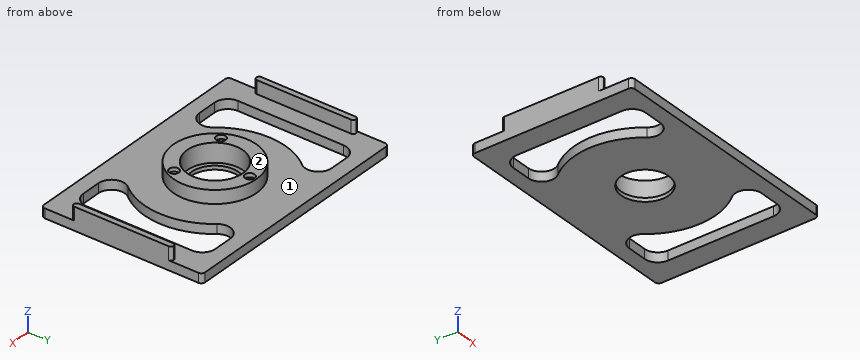
Autodesk Inventor part; units mm, degrees
ref_plane "YZ Plane" through (0, 0, 0) normal (1, 0, 0) x (0, 1, 0)
ref_plane "XZ Plane" through (0, 0, 0) normal (0, 1, 0) x (-1, 0, 0)
ref_plane "XY Plane" through (0, 0, 0) normal (0, 0, 1) x (1, 0, 0)
sketch "Skizze1" plane through (0, 0, 0) normal (0, 0, 1) x (1, 0, 0)
  line L0 (0, 0) -> (127.5, 0)
  line L1 (127.5, 0) -> (127.5, -85.5)
  line L2 (127.5, -85.5) -> (0, -85.5)
  line L3 (0, -85.5) -> (0, 0)
  dimension "d0" = 127.5
  dimension "d1" = 85.5
extrude "Extrusion1" add sketch "Skizze1" along normal blind 5
sketch "Skizze2" plane through (0, 0, 5) normal (0, 0, 1) x (1, 0, 0)
  line L0 (0, -16.25) -> (3, -16.25)
  line L1 (3, -16.25) -> (3, -69.25)
  line L2 (3, -69.25) -> (0, -69.25)
  line L3 (0, -69.25) -> (0, -16.25)
  line L4 (63.75, 42.9175) -> (63.75, -147.2432)
  line L5 (127.5, -85.5) -> (127.5, 0)
  line L6 (127.5, -16.25) -> (124.5, -16.25)
  line L7 (124.5, -16.25) -> (124.5, -69.25)
  line L8 (124.5, -69.25) -> (127.5, -69.25)
  line L9 (127.5, -69.25) -> (127.5, -16.25)
  point P0 (0, 0)
  dimension "d4" = 3
  dimension "d5" = 53
  dimension "d6" = 16.25
  dimension "d7" = 63.75
extrude "Extrusion2" add sketch "Skizze2" along normal blind 7
fillet "Rundung1" radius 2 4 edges at (0, 0, 2.5) (127.5, 0, 2.5) (127.5, -85.5, 2.5) (0, -85.5, 2.5)
fillet "Rundung2" radius 1.5 8 edges at (3, -69.25, 8.5) (0, -69.25, 8.5) (3, -16.25, 8.5) (0, -16.25, 8.5) (124.5, -16.25, 8.5) (127.5, -16.25, 8.5) (124.5, -69.25, 8.5) (127.5, -69.25, 8.5)
sketch "Skizze3" plane through (0, 0, 5) normal (0, 0, 1) x (1, 0, 0)
  circle A0 centre (63.75, -42.75) radius 12.5
  line L0 (0, -67.75) -> (0, -83.5)
  point P0 (0, 0)
  dimension "d12" = 25
  dimension "d13" = 63.75
  dimension "d14" = 42.75
extrude "Extrusion3" cut sketch "Skizze3" against normal blind 10
hole "Bohrung1" at (63.75, -42.75, 5) direction (0, 0, -1) diameter 29.5 depth 3
sketch "Skizze4" plane through (0, 0, 0) normal (0, 0, -1) x (-1, 0, 0)
  line L0 (-125.5, -85.5) -> (-2, -85.5)
  line L1 (0, -83.5) -> (0, -2)
  line L2 (-12, -77.75) -> (-50.2871, -77.75)
  line L3 (-50.2871, -7.75) -> (-12, -7.75)
  line L4 (-12, -7.75) -> (-12, -77.75)
  line L5 (-63.75, -42.75) -> (-63.75, -99.3052)
  line L6 (-115.5, -77.75) -> (-77.2129, -77.75)
  line L7 (-77.2129, -7.75) -> (-115.5, -7.75)
  line L8 (-115.5, -7.75) -> (-115.5, -77.75)
  arc A0 (-50.2871, -77.75) -> (-50.2871, -7.75) centre (-63.75, -42.75) ccw
  arc A1 (-77.2129, -7.75) -> (-77.2129, -77.75) centre (-63.75, -42.75) ccw
  arc A2 (-50.2871, -77.75) -> (-50.2871, -7.75) centre (-63.75, -42.75) ccw
  arc A3 (-77.2129, -7.75) -> (-77.2129, -77.75) centre (-63.75, -42.75) ccw
  point P0 (0, 0)
  dimension "d27" = 42.75
  dimension "d28" = 63.75
  dimension "d29" = 12
  dimension "d30" = 70
  dimension "d31" = 7.75
extrude "Extrusion4" cut sketch "Skizze4" against normal blind 10
fillet "Rundung3" radius 7 4 edges at (50.2871, -77.75, 2.5) (77.2129, -77.75, 2.5) (50.2871, -7.75, 2.5) (77.2129, -7.75, 2.5)
fillet "Rundung4" radius 7 4 edges at (12, -77.75, 2.5) (115.5, -77.75, 2.5) (12, -7.75, 2.5) (115.5, -7.75, 2.5)
sketch "Skizze5" plane through (0, 0, 5) normal (0, 0, 1) x (1, 0, 0)
  circle A0 centre (63.75, -42.75) radius 14.75
  circle A1 centre (63.75, -42.75) radius 22
  line L0 (125.5, 0) -> (2, 0)
  point P0 (0, 0)
  dimension "d36" = 29.5
  dimension "d37" = 44
  dimension "d38" = 42.75
  dimension "d39" = 63.75
extrude "Extrusion5" add sketch "Skizze5" along normal blind 7
sketch "Skizze6" plane through (63.75, -42.75, 12) normal (0, 0, 1) x (1, 0, 0)
  circle A0 centre (0, 18.5) radius 2.525
  circle A1 centre (0, 0) radius 12.5
  point P0 (-63.75, 42.75)
  dimension "d42" = 5.05
  dimension "d43" = 18.5
extrude "Extrusion6" cut sketch "Skizze6" against normal blind 2.1 contours A0
pattern_circular "Runde Anordnung1" count 3 over 360 about axis through (63.75, -42.75, 5) along (0, 0, 1) of "Extrusion6"
properties part number "Sensor Halterung293"
The listing builds one solid part. Answer for the finished solid, in the listing's coordinates (mm). Face numbers are marked on the shaded views. A direction names the side the tool comes from. Coordinates: 2 decimals unless noted, no trailing zeros. Loops run counter-clockwise (first coordinate to the right, second up) from the corner with the lowest first, then second, coordinate; pieces in that order, holes last. Notation, with made-up numbers: M -4,44 L 6,44 A35 cw 6,76 Z; hole C 35,-40 d2. An arc over 180 degrees is marked long. Answer in a Markdown table with one row per item.
1) Find the intervals of material crossed by probe 1 along X at (y, z) = (-42.5, 3); probe 2 along Y at (x, z) = (63.75, 0.95); probe 3 along X at (y, z) = (-42.5, 8.5), in increasing order.
Answers below:
| item | result |
|---|---|
| probe 1 | 0 to 12, 26.25 to 49, 78.5 to 101.25, 115.5 to 127.5 |
| probe 2 | -85.5 to -55.25, -30.25 to 0 |
| probe 3 | 0 to 3, 41.75 to 49, 78.5 to 85.75, 124.5 to 127.5 |
2) Find section D-D (y = -60). Determine the outline of the cut face in (x, z), then the cut area to 3 significant figures.
Answers below:
| item | result |
|---|---|
| outline | M 0,0 L 12,0 L 12,5 L 3,5 L 3,12 L 0,12 Z; M 30.45,0 L 97.05,0 L 97.05,5 L 77.4,5 L 77.4,12 L 50.1,12 L 50.1,5 L 30.45,5 Z; M 115.5,0 L 127.5,0 L 127.5,12 L 124.5,12 L 124.5,5 L 115.5,5 Z |
| area | 686 mm^2 |
3) Given pin 1 (6 mm diameter, centred on y = -74, z = 9.5, fed in from +X); pin 2 (4 mm diameter, centred on x = 84, z = 8.5, fed in from -Y); pin 3 (8 mm diameter, centred on x = 87.5, y = -55.5, fed in from +Z); pin 4 (1.5 mm diameter, centred on x = 64, y = -24, fed in from +Z), each flat-ended and moving along its own axis, determine where each tip first touches the part or whether it passes through.
Answers below:
| item | result |
|---|---|
| pin 1 | through |
| pin 2 | y = -55.04 |
| pin 3 | z = 5 |
| pin 4 | z = 9.9 |
4) Find section C-C (y = -42.75). Determine the outline of the cut face in (x, z), then the cut area to 3 significant figures.
Answers below:
| item | result |
|---|---|
| outline | M 0,0 L 12,0 L 12,5 L 3,5 L 3,12 L 0,12 Z; M 26.25,0 L 51.25,0 L 51.25,2 L 49,2 L 49,12 L 41.75,12 L 41.75,5 L 26.25,5 Z; M 76.25,0 L 101.25,0 L 101.25,5 L 85.75,5 L 85.75,12 L 78.5,12 L 78.5,2 L 76.25,2 Z; M 115.5,0 L 127.5,0 L 127.5,12 L 124.5,12 L 124.5,5 L 115.5,5 Z |
| area | 500 mm^2 |
5) Find section A-A (z = 6.75). Count the separate pieces of the cut face and the enclosed holes in it, then the cut area to 3 significant figures.
Answers below:
| item | result |
|---|---|
| separate pieces | 3 |
| enclosed holes | 1 |
| area | 1,150 mm^2 |
6) Which of the six approach directions +Z, -Z, +X, -X, +Y, -Y give full straight-line access (tool end or side, diameter ignored) to the marked faces 1 and 2?
Answers below:
| item | result |
|---|---|
| face 1 | +Z |
| face 2 | +Z, +X, -X, +Y, -Y |
7) Find section B-B (x = 63.75). Determine the outline of the cut face in (y, z) (3 decimals), then the cut area to 3 significant figures.
Answers below:
| item | result |
|---|---|
| outline | M -85.5,0 L -55.25,0 L -55.25,2 L -57.5,2 L -57.5,12 L -64.75,12 L -64.75,5 L -85.5,5 Z; M -30.25,0 L 0,0 L 0,5 L -20.75,5 L -20.75,12 L -21.725,12 L -21.725,9.9 L -26.775,9.9 L -26.775,12 L -28,12 L -28,2 L -30.25,2 Z |
| area | 380 mm^2 |
